Here's how the part is built. I have some questions about the finished solid (model axes, mm). Face numbers are marked on the shaded views. Round coordinates to 2 decimals unless told otherwise and drop trailing zeros. Order: outer loops, then holes, each group sorted by start corner. A loop starts at its lowest first (then second) coordinate and runs counter-clockwise, first axis right, second up. Notation, with made-up numbers: M -32,18.5 L -7,18.5 A19 cw -7,38.5 Z; hole C 30,54 d3. An arc over 180 degrees is marked long. Answer as CSV lines item,"result". Start each with the question number.
```python
from build123d import *

# Parameters (mm, degrees)
F0_R     = 12.7
F1_DEPTH = 6.35
F2_R     = 10.16
F3_DEPTH = 6.35
F4_R     = 6.35
F5_DEPTH = 50.8
F6_R     = 8.89
F7_DEPTH = 5.08
F9_DEPTH = 279.4


with BuildPart() as f1:
    # F0 (on Front) → F1 (new body)
    with BuildSketch(Plane.XZ):
        with Locations((-96.856251, 20.265313)):
            Circle(F0_R)
    extrude(amount=-F1_DEPTH)

    # F2 (on face) → F3 (join)
    with BuildSketch(Plane(origin=(0, 6.35, 0), x_dir=(-1, 0, 0), z_dir=(0, 1, 0))):
        with Locations((96.856251, 20.265313)):
            Circle(F2_R)
    extrude(amount=F3_DEPTH)

    # F4 (on face) → F5 (join)
    with BuildSketch(Plane(origin=(0, 12.7, 0), x_dir=(-1, 0, 0), z_dir=(0, 1, 0))):
        with Locations((96.856251, 20.265313)):
            Circle(F4_R)
    extrude(amount=F5_DEPTH)

    # F6 (on face) → F7 (join)
    with BuildSketch(Plane(origin=(0, 63.5, 0), x_dir=(-1, 0, 0), z_dir=(0, 1, 0))):
        with Locations((96.856251, 20.265313)):
            Circle(F6_R)
    extrude(amount=F7_DEPTH)

    # F8 (on face) → F9 (join)
    with BuildSketch(Plane.XZ):
        Polygon((-96.659377, 28.0142), (-102.123946, 11.775506), (-91.156051, 11.775506), align=None)
    extrude(amount=F9_DEPTH)


solid = f1.part
```
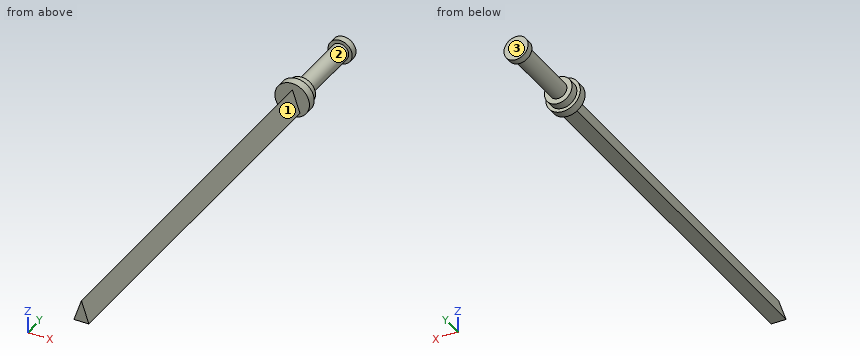
Item 1: If we section it at B-B on y = 20.5: Please give me the cut outline in (x, z).
Item 2: If we section it at A-A on y = -163.5: Please give me the cut outline in (x, z).
Item 3: We'd pull the mould along Y, two halves only. Please class the marked faces 1, 2 and 3: pulls with the +Y half, pulls with the -Y half, needs draft (parallel to the pull), parting line crosses it, or undercut.
Item 4: For P1, Ø12, axis at x = -100.5, y = -78, coming from the -Z side; P2, Ø12, axis at y = -196.5, z = 30, coming from the -X side; P3, Ø1, axis at y = 27, z = 18.5, coming from the +X side, each with a flat end and sliding along its axis, tell me the tip position at first contact or that it passes through.
Item 5: If I drill on line 1 along Y through (x, z) = (-90, 16.75); line 2 along Y through (x, z) = (-100.5, 17.5); line 3 along Y through (x, z) = (-92.75, 11.5), over which ranges is the centre line in solid material (lowest first)?
Geometry says:
1,outline,"C -96.86,20.27 d12.7"
2,outline,"M -102.12,11.78 L -91.16,11.78 L -96.66,28.01 Z"
3,face 1,"needs draft"
3,face 2,"undercut"
3,face 3,"pulls with the +Y half"
4,P1,"z = 11.78"
4,P2,"x = -98.01"
4,P3,"x = -90.63"
5,line 1,"0 to 12.7, 63.5 to 68.58"
5,line 2,"0 to 68.58"
5,line 3,"0 to 12.7"
